Source: CAD feature listing. Evaluate the final solid. Frame: model axes, mm. A direction names the side the tool comes from. Give positions to 0.01 mm unless a question says otherwise; leave off trailing zeros.
from build123d import *

# Parameters (mm, degrees)
SKETCH011_W     = 60.3
SKETCH011_H     = 32.3
PAD003_DEPTH    = 4.5
PAD003_TAPER    = 40
FILLET001_R     = 2
PAD004_DEPTH    = 0.5
PAD005_DEPTH    = 0.4
SKETCH014_R     = 2
POCKET008_DEPTH = 2
SKETCH015_R     = 2
POCKET009_DEPTH = 1
POCKET009_TAPER = 17.5


with BuildPart() as part:
    # Sketch011 → Pad003 (new body)
    with BuildSketch(Plane.XY):
        with Locations((-2.81, -16.15)):
            Rectangle(SKETCH011_W, SKETCH011_H)
    extrude(amount=-PAD003_DEPTH, taper=PAD003_TAPER)

    # Fillet001
    fillet001_edges = [part.edges().sort_by_distance(p)[0] for p in [
        (-29.184052, -16.15, -4.5),
        (-31.072026, -1.887974, -2.25),
        (-2.81, -3.775948, -4.5),
        (-2.81, -28.524052, -4.5),
        (25.452026, -1.887974, -2.25),
        (23.564052, -16.15, -4.5),
        (25.452026, -30.412026, -2.25),
        (-31.072026, -30.412026, -2.25),
    ]]
    fillet(fillet001_edges, radius=FILLET001_R)

    # Sketch012 (on Face13 of Fillet001) → Pad004 (join)
    with BuildSketch(Plane(origin=(0, 0, -4.5), x_dir=(1, 0, 0), z_dir=(0, 0, -1))):
        with BuildLine():
            Line((4.381436, 25.091436), (4.381436, 21.591436))
            ThreePointArc((4.381436, 21.591436), (4.527883, 21.237883), (4.881436, 21.091436))
            Line((4.881436, 21.091436), (16.631436, 21.091436))
            ThreePointArc((16.631436, 21.091436), (16.98499, 21.237883), (17.131436, 21.591436))
            Line((17.131436, 21.591436), (17.131436, 25.091436))
            ThreePointArc((17.131436, 25.091436), (16.98499, 25.44499), (16.631436, 25.591436))
            Line((16.631436, 25.591436), (4.881436, 25.591436))
            ThreePointArc((4.881436, 25.591436), (4.527883, 25.44499), (4.381436, 25.091436))
        make_face()
        with BuildLine():
            Line((4.381436, 10.708564), (4.381436, 7.208564))
            ThreePointArc((4.381436, 7.208564), (4.527883, 6.85501), (4.881436, 6.708564))
            Line((4.881436, 6.708564), (16.631436, 6.708564))
            ThreePointArc((16.631436, 6.708564), (16.98499, 6.85501), (17.131436, 7.208564))
            Line((17.131436, 7.208564), (17.131436, 10.708564))
            ThreePointArc((17.131436, 10.708564), (16.98499, 11.062117), (16.631436, 11.208564))
            Line((16.631436, 11.208564), (4.881436, 11.208564))
            ThreePointArc((4.881436, 11.208564), (4.527883, 11.062117), (4.381436, 10.708564))
        make_face()
        with BuildLine():
            Line((-27.351436, 22.025), (-27.351436, 10.275))
            ThreePointArc((-27.351436, 10.275), (-27.20499, 9.921447), (-26.851436, 9.775))
            Line((-26.851436, 9.775), (-23.351436, 9.775))
            ThreePointArc((-23.351436, 9.775), (-22.997883, 9.921447), (-22.851436, 10.275))
            Line((-22.851436, 10.275), (-22.851436, 22.025))
            ThreePointArc((-22.851436, 22.025), (-22.997883, 22.378553), (-23.351436, 22.525))
            Line((-23.351436, 22.525), (-26.851436, 22.525))
            ThreePointArc((-26.851436, 22.525), (-27.20499, 22.378553), (-27.351436, 22.025))
        make_face()
    extrude(amount=PAD004_DEPTH)

    # Sketch013 (on Face45 of Pad004) → Pad005 (join)
    with BuildSketch(Plane(origin=(0, 0, -5), x_dir=(1, 0, 0), z_dir=(0, 0, -1))):
        with BuildLine():
            Line((4.781436, 24.941436), (4.781436, 21.741436))
            ThreePointArc((4.781436, 21.741436), (4.85466, 21.56466), (5.031436, 21.491436))
            Line((5.031436, 21.491436), (16.481436, 21.491436))
            ThreePointArc((16.481436, 21.491436), (16.658213, 21.56466), (16.731436, 21.741436))
            Line((16.731436, 21.741436), (16.731436, 24.941436))
            ThreePointArc((16.731436, 24.941436), (16.658213, 25.118213), (16.481436, 25.191436))
            Line((16.481436, 25.191436), (5.031436, 25.191436))
            ThreePointArc((5.031436, 25.191436), (4.85466, 25.118213), (4.781436, 24.941436))
        make_face()
        with BuildLine():
            Line((4.781436, 10.558564), (4.781436, 7.358564))
            ThreePointArc((4.781436, 7.358564), (4.85466, 7.181787), (5.031436, 7.108564))
            Line((5.031436, 7.108564), (16.481436, 7.108564))
            ThreePointArc((16.481436, 7.108564), (16.658213, 7.181787), (16.731436, 7.358564))
            Line((16.731436, 7.358564), (16.731436, 10.558564))
            ThreePointArc((16.731436, 10.558564), (16.658213, 10.73534), (16.481436, 10.808564))
            Line((16.481436, 10.808564), (5.031436, 10.808564))
            ThreePointArc((5.031436, 10.808564), (4.85466, 10.73534), (4.781436, 10.558564))
        make_face()
        with BuildLine():
            Line((-26.951436, 21.875), (-26.951436, 10.425))
            ThreePointArc((-26.951436, 10.425), (-26.878213, 10.248223), (-26.701436, 10.175))
            Line((-26.701436, 10.175), (-23.501436, 10.175))
            ThreePointArc((-23.501436, 10.175), (-23.32466, 10.248223), (-23.251436, 10.425))
            Line((-23.251436, 10.425), (-23.251436, 21.875))
            ThreePointArc((-23.251436, 21.875), (-23.32466, 22.051777), (-23.501436, 22.125))
            Line((-23.501436, 22.125), (-26.701436, 22.125))
            ThreePointArc((-26.701436, 22.125), (-26.878213, 22.051777), (-26.951436, 21.875))
        make_face()
    extrude(amount=PAD005_DEPTH)

    # Sketch014 → Pocket008 (cut)
    with BuildSketch(Plane.XY):
        with Locations((-22.41, -10.45)):
            Circle(SKETCH014_R)
        with Locations((-22.41, -21.85)):
            Circle(SKETCH014_R)
    extrude(amount=-POCKET008_DEPTH, mode=Mode.SUBTRACT)

    # Sketch015 → Pocket009 (cut)
    with BuildSketch(Plane.XY):
        with Locations((24.59, -10.45)):
            Circle(SKETCH015_R)
        with Locations((24.59, -21.85)):
            Circle(SKETCH015_R)
    extrude(amount=-POCKET009_DEPTH, taper=POCKET009_TAPER, mode=Mode.SUBTRACT)


with BuildPart() as part_1:
    # Body002 placement: moved
    add(part.part.moved(Location((0, -30.35, 0))))


solid = part_1.part
1) Reachability of faces 1 (the face through (11.2, -55.7, -5)), 2 (the face through (-25, -47, -5.4)), 3 (the face through (25, -52, -1)) from +Z, -Z, +X, -X, +Y, -Y: full face, straight path, thin tool, end or side. Return the list, or none.
Checks:
face 1: -Z
face 2: -Z, +X, -X, +Y, -Y
face 3: +Z
2) Ray query, L1, parallel to Y at x = -22.41, z = -1.4; L2, parallel to Y at x = -22.41, z = -1.5; L3, parallel to Z at x = 12.5, y = -48. Return the intervals inside material, ascending.
Checks:
L1: y = -61.48 to -54.2, -50.2 to -42.8, -38.8 to -31.52
L2: y = -61.39 to -54.2, -50.2 to -42.8, -38.8 to -31.61
L3: z = -4.5 to 0
3) Pull-direction query (X, two-part tool) for faces 4 (the face through (11, -54, -5.4)), 5 (the face through (-22.67, -50.217, -0.986)), 6 (the face through (-22, -41, -2)); classes: +X half, -X half, draft (parallel to the pull), parting line (faces both ways), or undercut.
Checks:
face 4: draft
face 5: undercut
face 6: undercut
4) First-contact query: pin 1 Ø3 at (x, z) = (-26, -3) entering from -Y; pin 2 Ø3 at (y, z) = (-49, -4) entering from +X; pin 3 Ø2 at (x, y) = (4, -50) entering from -Z. Flat tips, straight axial feed; report the tip coordinate or a pass-through.
Checks:
pin 1: stops at y = -61.39
pin 2: stops at x = 25.24
pin 3: stops at z = -4.5
